Read the model definition and answer for the solid it produces. Units are mm, in the model's axes. Face numbers are marked on the shaded views. A direction names the side the tool comes from. Coordinates: 2 decimals unless noted, no trailing zeros. Loops run counter-clockwise (first coordinate to the right, second up) from the corner with the lowest first, then second, coordinate; pieces in that order, holes last.
Q1. Flat-ended cylindrical pins translate along their axes: P1, Ø2, axis at x = 10.5, z = -42.5, coming from the +Y side; P2, Ø1.2, axis at y = 28, z = 2.5, coming from the -X side; P3, Ø2.5, axis at y = 35, z = -12.5, coming from the +X side. Find the tip coordinate at first contact, or state that the pin passes through.
Q2. Straight lines are drawn through the part: line 1 (X direction, y = 28.1, z = -43.6); line 2 (Z direction, x = 4.8, y = 27.9); line 3 (Y direction, x = 6, z = 1). For each, find the intervals that lie inside material, in ascending order.
Q3. Section B-B (x = 6.25) is taken. Count the separate pieces of the cut face and the enclosed holes in it, then the cut area to 3 significant figures.
Q4. Section D-D (z = -18.5) is taken. Give the vertices of the cut face in (x, y), then the cut area to 3 significant figures.
Q5. Which of the six approach directions +Z, -Z, +X, -X, +Y, -Y give full straight-line access (tool end or side, diameter ignored) to the marked faces 1 and 2?
Q6. Section C-C (y = 35) is taken. Give the vertices of the cut face in (x, z), then the cut area to 3 significant figures.
Q7. Section A-A (z = -30.45) is taken. Give the vertices of the cut face in (x, y).
from build123d import *

# Parameters (mm, degrees)
SKETCH1_W                = 20
SKETCH1_H                = 40
BOSS_EXTRUDE1_DEPTH      = 33.3
SKETCH2_W                = 19
SKETCH2_H                = 2.5
BOSS_EXTRUDE2_DEPTH      = 6.6
SKETCH3_W                = 19
SKETCH3_H                = 2.5
BOSS_EXTRUDE3_DEPTH      = 6.6
SKETCH4_R                = 9.55
BOSS_EXTRUDE4_DEPTH      = 3
SKETCH12_W               = 18.4
SKETCH12_H               = 26
BOSS_EXTRUDE10_DEPTH     = 3
SKETCH11_R               = 0.5
BOSS_EXTRUDE9_DEPTH      = 3
LPATTERN2_COUNT          = 3
LPATTERN2_PITCH          = 1.01
SKETCH13_R               = 6.45
BOSS_EXTRUDE11_DEPTH     = 1.6
SKETCH14_R               = 5
BOSS_EXTRUDE12_DEPTH     = 0.5
SKETCH15_R               = 3
BOSS_EXTRUDE13_DEPTH     = 3.3
BOSS_EXTRUDE14_DEPTH     = 3
SKETCH17_W               = 1.3
SKETCH17_H               = 3.8
BOSS_EXTRUDE15_DEPTH     = 0.9
SKETCH18_W               = 1.3
SKETCH18_H               = 3.8
BOSS_EXTRUDE16_DEPTH     = 0.9
M4_CLEARANCE_HOLE1_D     = 4.5
M4_CLEARANCE_HOLE1_DEPTH = 3
M4_CLEARANCE_HOLE1_TIP   = 1.351936393


with BuildPart() as part:
    # Sketch1 → Boss-Extrude1 (new body)
    with BuildSketch(Plane(origin=(0, 0, 0), x_dir=(1, 0, 0), z_dir=(0, 1, 0))):
        with Locations((10, 20)):
            Rectangle(SKETCH1_W, SKETCH1_H)
    extrude(amount=BOSS_EXTRUDE1_DEPTH)

    # Sketch2 → Boss-Extrude2 (add)
    with BuildSketch(Plane.XY):
        with Locations((10, 27.75)):
            Rectangle(SKETCH2_W, SKETCH2_H)
    extrude(amount=BOSS_EXTRUDE2_DEPTH)

    # Sketch3 → Boss-Extrude3 (add)
    with BuildSketch(Plane(origin=(0, 0, -40), x_dir=(-1, 0, 0), z_dir=(0, 0, -1))):
        with Locations((-10, 27.75)):
            Rectangle(SKETCH3_W, SKETCH3_H)
    extrude(amount=BOSS_EXTRUDE3_DEPTH)

    # Sketch4 → Boss-Extrude4 (add)
    with BuildSketch(Plane(origin=(0, 33.3, 0), x_dir=(1, 0, 0), z_dir=(0, 1, 0))):
        with Locations(Location((10, 30.45, 0), (0, 0, 90))):
            Circle(SKETCH4_R)
    extrude(amount=BOSS_EXTRUDE4_DEPTH)

    # Sketch12 → Boss-Extrude10 (add)
    with BuildSketch(Plane(origin=(0, 33.3, 0), x_dir=(1, 0, 0), z_dir=(0, 1, 0))):
        with Locations((10, 17.9)):
            Rectangle(SKETCH12_W, SKETCH12_H)
    extrude(amount=BOSS_EXTRUDE10_DEPTH)

    # Sketch11 → Boss-Extrude9 (add)
    with BuildSketch(Plane(origin=(0, 0, -40), x_dir=(-1, 0, 0), z_dir=(0, 0, -1))):
        with Locations(Location((-11.2, 2.4, 0), (0, 0, 180))):
            Circle(SKETCH11_R)
    boss_extrude9 = extrude(amount=BOSS_EXTRUDE9_DEPTH)

    # LPattern2: Boss-Extrude9 ×3
    with Locations(*[(-i * LPATTERN2_PITCH, 0, 0) for i in range(1, LPATTERN2_COUNT)]):
        add(boss_extrude9)

    # Sketch13 → Boss-Extrude11 (add)
    with BuildSketch(Plane(origin=(0, 36.3, 0), x_dir=(1, 0, 0), z_dir=(0, 1, 0))):
        with Locations(Location((10, 30.45, 0), (0, 0, 270))):
            Circle(SKETCH13_R)
    extrude(amount=BOSS_EXTRUDE11_DEPTH)

    # Sketch14 → Boss-Extrude12 (add)
    with BuildSketch(Plane(origin=(0, 37.9, 0), x_dir=(1, 0, 0), z_dir=(0, 1, 0))):
        with Locations(Location((10, 30.45, 0), (0, 0, 270))):
            Circle(SKETCH14_R)
    extrude(amount=BOSS_EXTRUDE12_DEPTH)

    # Sketch15 → Boss-Extrude13 (add)
    with BuildSketch(Plane(origin=(0, 38.4, 0), x_dir=(1, 0, 0), z_dir=(0, 1, 0))):
        with Locations(Location((10, 30.45, 0), (0, 0, 270))):
            Circle(SKETCH15_R)
    extrude(amount=BOSS_EXTRUDE13_DEPTH)

    # Sketch16 → Boss-Extrude14 (add)
    with BuildSketch(Plane(origin=(0, 33.3, 0), x_dir=(1, 0, 0), z_dir=(0, 1, 0))):
        with BuildLine():
            Line((14.4, 4.9), (5.6, 4.9))
            ThreePointArc((5.6, 4.9), (10, 2.9), (14.4, 4.9))
        make_face()
    extrude(amount=BOSS_EXTRUDE14_DEPTH)

    # Sketch17 → Boss-Extrude15 (add)
    with BuildSketch(Plane(origin=(0, 29, 0), x_dir=(1, 0, 0), z_dir=(0, 1, 0))):
        with Locations((10, -1.9)):
            Rectangle(SKETCH17_W, SKETCH17_H)
    extrude(amount=BOSS_EXTRUDE15_DEPTH)

    # Sketch18 → Boss-Extrude16 (add)
    with BuildSketch(Plane(origin=(0, 29, 0), x_dir=(1, 0, 0), z_dir=(0, 1, 0))):
        with Locations((10, 41.9)):
            Rectangle(SKETCH18_W, SKETCH18_H)
    extrude(amount=BOSS_EXTRUDE16_DEPTH)

    # M4 Clearance Hole1
    with Locations(Plane(origin=(0, 29, 0), x_dir=(1, 0, 0), z_dir=(0, 1, 0))):
        with Locations((4.8, 43.6), (15.2, 43.6), (4.8, -3.6), (15.2, -3.6)):
            Hole(M4_CLEARANCE_HOLE1_D / 2, depth=M4_CLEARANCE_HOLE1_DEPTH)
            with Locations((0, 0, -(M4_CLEARANCE_HOLE1_DEPTH + M4_CLEARANCE_HOLE1_TIP / 2))):  # 118° drill point
                Cone(0, M4_CLEARANCE_HOLE1_D / 2, M4_CLEARANCE_HOLE1_TIP, mode=Mode.SUBTRACT)


solid = part.part
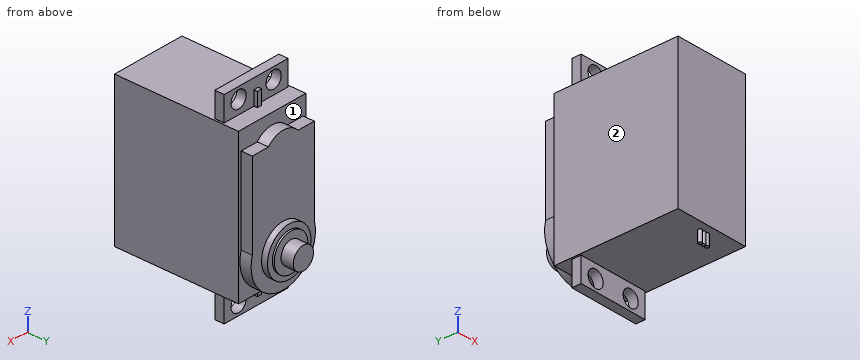
Numbers:
1. P1: stops at y = 29.9
1. P2: stops at x = 0.5
1. P3: stops at x = 19.2
2. line 1: x = 0.5 to 2.55, 7.05 to 12.95, 17.45 to 19.5
2. line 2: z = -46.6 to -45.85, -41.35 to 1.35, 5.85 to 6.6
2. line 3: y = 26.5 to 29
3. separate pieces: 3
3. enclosed holes: 0
3. area: 1,470 mm2
4. outline: (0, 0) - (20, 0) - (20, 33.3) - (19.2, 33.3) - (19.2, 36.3) - (0.8, 36.3) - (0.8, 33.3) - (0, 33.3) - close
4. area: 721 mm2
5. face 1: +Y
5. face 2: +Z, -Z, -X, +Y, -Y
6. outline: (0.8, -27.89) arc R9.55 ccw (long way) to (19.2, -27.89) - (19.2, -4.9) - (14.4, -4.9) arc R5.84 ccw to (5.6, -4.9) - (0.8, -4.9) - close
6. area: 627 mm2
7. outline: (0, 0) - (20, 0) - (20, 33.3) - (19.55, 33.3) - (19.55, 36.3) - (16.45, 36.3) - (16.45, 37.9) - (15, 37.9) - (15, 38.4) - (13, 38.4) - (13, 41.7) - (7, 41.7) - (7, 38.4) - (5, 38.4) - (5, 37.9) - (3.55, 37.9) - (3.55, 36.3) - (0.45, 36.3) - (0.45, 33.3) - (0, 33.3) - close
